Build history of the part. All positions in model axes, mm. A direction names the side the tool comes from. Give positions to 0.01 mm unless a question says otherwise; leave off trailing zeros. Loops run counter-clockwise (first coordinate to the right, second up) from the corner with the lowest first, then second, coordinate; pieces in that order, holes last. Notation, with made-up numbers: M 16.25,79.5 L 67.25,79.5 A27 ccw 67.25,102.5 Z; hole C 3.5,39 d2. An arc over 180 degrees is marked long. Answer in a Markdown table with one row per item. Add a question column.
```python
from build123d import *

# Parameters (mm, degrees)
SKETCH_W        = 80
SKETCH_H        = 80
PAD_DEPTH       = 4
SKETCH001_R     = 1.5
PAD001_DEPTH    = 25
FILLET_R        = 20
CHAMFER_SIZE    = 2
CHAMFER001_SIZE = 0.5
CHAMFER002_SIZE = 1


with BuildPart() as part:
    # Sketch → Pad (new body)
    with BuildSketch(Plane.XY):
        with Locations((40, 40)):
            Rectangle(SKETCH_W, SKETCH_H)
    extrude(amount=PAD_DEPTH)

    # Sketch001 → Pad001 (new body)
    with BuildSketch(Plane.XY.offset(4)):
        with Locations((60, 60)):
            Circle(SKETCH001_R)
        with Locations((20, 60)):
            Circle(SKETCH001_R)
        with Locations((20, 20)):
            Circle(SKETCH001_R)
        with Locations((60, 20)):
            Circle(SKETCH001_R)
    extrude(amount=PAD001_DEPTH)

    # Fillet
    fillet_edges = [part.edges().sort_by_distance(p)[0] for p in [
        (80, 0, 2),
        (80, 80, 2),
        (0, 0, 2),
        (0, 80, 2),
    ]]
    fillet(fillet_edges, radius=FILLET_R)

    # Chamfer
    chamfer_edges = [part.edges().sort_by_distance(p)[0] for p in [
        (58.5, 20, 4),
        (18.5, 20, 4),
        (18.5, 60, 4),
        (58.5, 60, 4),
    ]]
    chamfer(chamfer_edges, length=CHAMFER_SIZE)

    # Chamfer001
    chamfer001_edges = [part.edges().sort_by_distance(p)[0] for p in [
        (40, 80, 0),
        (5.857864, 74.142136, 0),
        (74.142136, 74.142136, 0),
        (0, 40, 0),
        (80, 40, 0),
        (5.857864, 5.857864, 0),
        (74.142136, 5.857864, 0),
        (40, 0, 0),
    ]]
    chamfer(chamfer001_edges, length=CHAMFER001_SIZE)

    # Chamfer002
    chamfer002_edges = [part.edges().sort_by_distance(p)[0] for p in [
        (74.142136, 5.857864, 4),
        (80, 40, 4),
        (74.142136, 74.142136, 4),
        (40, 80, 4),
        (5.857864, 74.142136, 4),
        (0, 40, 4),
        (5.857864, 5.857864, 4),
        (40, 0, 4),
    ]]
    chamfer(chamfer002_edges, length=CHAMFER002_SIZE)


solid = part.part
```
(1) Pull direction Y, two halves, no side cores. Call faces 3 (the cylindrical face through (18.89, 21.01, 17.34)), 4 (the flat face through (0, 40, 2)), 5 (the conical face through (5.96, 73.73, 0.14)): +Y half, -Y half, draft (parallel to the pull), parting line (faces both ways), or undercut.
(2) Slice it at A-A, the plane y = 36. Give the cut face in (x, z), then the cut area to 3 significant figures.
(3) Wall check: line 1 (Y direction, x = 60, z = 13.5); line 2 (Z direction, x = 35.5, y = 5); line 3 (X direction, y = 65.5, z = 2.25). Give the ranges that are in metal, low to high.
(4) Slice it at C-C, the plane z = 25.5. Give the cut face in (x, y).
(5) Pin check, flat tips, straight feed: pin 1 (8 mm diameter, centred on y = 50.5, z = 3.5, fed in from +X); pin 2 (1 mm diameter, centred on y = 20, z = 15.5, fed in from +X). Stop position of each tip, or through.
(6) Tool access for faces 1 (the cylindrical face through (18.89, 61.01, 17.34)), 2 (the flat face through (60, 20, 29)): list every direction of +Z, -Z, +X, -X, +Y, -Y with a clear straight run to the whole face (end or side of a thin tool).
Solution:
| question | item | result |
|---|---|---|
| 1 | face 3 | undercut |
| 1 | face 4 | draft |
| 1 | face 5 | +Y half |
| 2 | outline | M 0,0.5 L 0.5,0 L 79.5,0 L 80,0.5 L 80,3 L 79,4 L 1,4 L 0,3 Z |
| 2 | area | 319 mm^2 |
| 3 | line 1 | 18.5 to 21.5, 58.5 to 61.5 |
| 3 | line 2 | 0 to 4 |
| 3 | line 3 | 0.77 to 79.23 |
| 4 | outline | C 20,20 d3; C 20,60 d3; C 60,20 d3; C 60,60 d3 |
| 5 | pin 1 | x = 80 |
| 5 | pin 2 | x = 61.5 |
| 6 | face 1 | +Z |
| 6 | face 2 | +Z, +X, -X, +Y, -Y |
